Geometry: final body of the model. Coordinates: model frame, mm. Give positions to 0.01 mm unless a question says otherwise; leave off trailing zeros. Order: outer loops, then holes, each group sorted by start corner. A loop starts at its lowest first (then second) coordinate and runs counter-clockwise, first axis right, second up. Notation, with made-up numbers: (61.5, 87) -> (107.5, 87) arc R14 cw to (107.5, 113) -> close; hole circle Ø8 at (50.5, 62.5). An arc over 180 degrees is marked (long way). Answer in a Markdown table with one row per item. Add a question column.
Q1. Pull-direction query (Z, two-part tool) for faces 1 (the face through (-2.96, 10.84, -9.42)), 2 (the face through (-3, 18, 39)), 3 (the face through (0, -4, 1)); classes: +Z half, -Z half, draft (parallel to the pull), parting line (faces both ways), or undercut.
Q2. Cut plane A-A on z = -32. Return the cut outline in (x, y).
Q3. Cut plane D-D on x = -1.3. Return the cut outline in (y, z).
Q4. Line query: line 1 along Y through (x, z) = (-2.05, 0); line 2 along Z through (x, y) = (-4.5, 1); line 3 along Z through (x, y) = (-1.25, 11.5). Output: solid intervals per line, ascending. Write a range as from..to.
Q5. Cut plane B-B on y = -6. Return the cut outline in (x, z).
Q6. Contact query for a flat-ended pin moving along its axis: P1, Ø5.5, axis at y = -6, z = 32, coming from the +X side. Output: stop coordinate, or through.
Q7. Cut plane C-C on z = -10. Return the cut outline in (x, y).
from build123d import *

# Parameters (mm, degrees)
SKETCH3_W           = 80
SKETCH3_H           = 40
BOSS_EXTRUDE3_DEPTH = 6
SKETCH4_R           = 5
SKETCH4_R_2         = 1.5
SKETCH4_R_3         = 3.4
CUT_EXTRUDE1_DEPTH  = 8
FILLET1_R           = 5


with BuildPart() as part:
    # Sketch3 → Boss-Extrude3 (new body)
    with BuildSketch(Plane(origin=(0, 0, 0), x_dir=(0, 0, -1), z_dir=(1, 0, 0))):
        Rectangle(SKETCH3_W, SKETCH3_H)
    extrude(amount=-BOSS_EXTRUDE3_DEPTH)

    # Sketch4 → Cut-Extrude1 (cut)
    with BuildSketch(Plane(origin=(0, 0, 0), x_dir=(0, 0, -1), z_dir=(1, 0, 0))):
        with Locations((0, 1.15)):
            Circle(SKETCH4_R)
        with Locations((-10.606601718, 11.756601718)):
            Circle(SKETCH4_R_2)
        with Locations((10.606601718, 11.756601718)):
            Circle(SKETCH4_R_2)
        with Locations((10.606601718, -9.456601718)):
            Circle(SKETCH4_R_2)
        with Locations((-10.606601718, -9.456601718)):
            Circle(SKETCH4_R_2)
        with Locations((32, -6)):
            Circle(SKETCH4_R_3)
        with Locations((-32, -6)):
            Circle(SKETCH4_R_3)
    extrude(amount=-CUT_EXTRUDE1_DEPTH, mode=Mode.SUBTRACT)

    # Fillet1
    fillet1_edges = [part.edges().sort_by_distance(p)[0] for p in [
        (-3, 20, 40),
        (-3, 20, -40),
    ]]
    fillet(fillet1_edges, radius=FILLET1_R)


solid = part.part
Completed:
| question | item | result |
|---|---|---|
| 1 | face 1 | undercut |
| 1 | face 2 | +Z half |
| 1 | face 3 | draft |
| 2 | outline | (-6, -20) -> (0, -20) -> (0, -9.4) -> (-6, -9.4) -> close; (-6, -2.6) -> (0, -2.6) -> (0, 20) -> (-6, 20) -> close |
| 3 | outline | (-20, -40) -> (15, -40) arc R5 ccw to (20, -35) -> (20, 35) arc R5 ccw to (15, 40) -> (-20, 40) -> close; hole circle Ø3 at (-9.46, -10.61); hole circle Ø3 at (-9.46, 10.61); hole circle Ø6.8 at (-6, -32); hole circle Ø6.8 at (-6, 32); hole circle Ø10 at (1.15, 0); hole circle Ø3 at (11.76, -10.61); hole circle Ø3 at (11.76, 10.61) |
| 4 | line 1 | y = -20..-3.85, 6.15..20 |
| 4 | line 2 | z = -40..-5, 5..40 |
| 4 | line 3 | z = -40..-12.08, -9.13..9.13, 12.08..40 |
| 5 | outline | (-6, -40) -> (0, -40) -> (0, -35.4) -> (-6, -35.4) -> close; (-6, -28.6) -> (0, -28.6) -> (0, 28.6) -> (-6, 28.6) -> close; (-6, 35.4) -> (0, 35.4) -> (0, 40) -> (-6, 40) -> close |
| 6 | P1 | passes through |
| 7 | outline | (-6, -20) -> (0, -20) -> (0, -10.83) -> (-6, -10.83) -> close; (-6, -8.08) -> (0, -8.08) -> (0, 10.38) -> (-6, 10.38) -> close; (-6, 13.13) -> (0, 13.13) -> (0, 20) -> (-6, 20) -> close |
